Can you work these out from the model? Positions are in its coordinate system, mm. Face numbers are marked on the shaded views. A direction names the side the tool comes from. Give positions to 0.01 mm unless a question says otherwise; leave off trailing zeros. Loops run counter-clockwise (first coordinate to the right, second up) from the corner with the lowest first, then second, coordinate; pieces in that order, holes last. Notation, with made-up numbers: (-12, -20) - (33, -20) arc R19 ccw to (33, -12) - close; hole circle Ø9 at (29, 62). An arc over 180 degrees is marked (long way). Answer in a Markdown table with one row per item.
from build123d import *

# Parameters (mm, degrees)
SKETCH1_W           = 203.2
SKETCH1_H           = 304.8
BOSS_EXTRUDE1_DEPTH = 203.2
SKETCH2_W           = 177.8
SKETCH2_H           = 279.4
CUT_EXTRUDE1_DEPTH  = 190.5
SKETCH3_W           = 7.62
SKETCH3_H           = 101.6
CUT_EXTRUDE2_DEPTH  = 190.5
SKETCH4_R           = 6.35
BOSS_EXTRUDE2_DEPTH = 279.4
BOSS_EXTRUDE3_DEPTH = 25.4
CUT_EXTRUDE3_DEPTH  = 12.7
SKETCH4_2_R         = 6.35
BOSS_EXTRUDE5_DEPTH = 12.7


with BuildPart() as part:
    # Sketch1 → Boss-Extrude1 (new body)
    with BuildSketch(Plane.XY):
        Rectangle(SKETCH1_W, SKETCH1_H)
    extrude(amount=BOSS_EXTRUDE1_DEPTH)

    # Sketch2 → Cut-Extrude1 (cut)
    with BuildSketch(Plane.XY.offset(203.2)):
        Rectangle(SKETCH2_W, SKETCH2_H)
    extrude(amount=-CUT_EXTRUDE1_DEPTH, mode=Mode.SUBTRACT)

    # Sketch3 → Cut-Extrude2 (cut)
    with BuildSketch(Plane(origin=(0, 152.4, 0), x_dir=(1, 0, 0), z_dir=(0, 1, 0))):
        with Locations((0, -101.6)):
            Rectangle(SKETCH3_W, SKETCH3_H)
    extrude(amount=-CUT_EXTRUDE2_DEPTH, mode=Mode.SUBTRACT)

    # Sketch4 → Boss-Extrude2 (add)
    with BuildSketch(Plane(origin=(0, -139.7, 0), x_dir=(1, 0, 0), z_dir=(0, 1, 0))):
        with Locations((-69.85, -63.5)):
            Circle(SKETCH4_R)
        with Locations((69.85, -63.5)):
            Circle(SKETCH4_R)
        with Locations((69.85, -139.7)):
            Circle(SKETCH4_R)
        with Locations((-69.85, -139.7)):
            Circle(SKETCH4_R)
    extrude(amount=BOSS_EXTRUDE2_DEPTH)

    # Sketch7 → Boss-Extrude3 (add)
    with BuildSketch(Plane(origin=(0, -139.7, 0), x_dir=(1, 0, 0), z_dir=(0, 1, 0))):
        with BuildLine():
            Line((-69.85, -53.975), (-60.325, -53.975))
            Line((-60.325, -53.975), (-28.575, -53.975))
            Line((-28.575, -53.975), (-28.575, -149.225))
            Line((-28.575, -149.225), (-60.325, -149.225))
            Line((-60.325, -149.225), (-69.85, -149.225))
            ThreePointArc((-69.85, -149.225), (-79.375, -139.7), (-69.85, -130.175))
            Line((-69.85, -130.175), (-60.325, -130.175))
            Line((-60.325, -130.175), (-60.325, -73.025))
            Line((-60.325, -73.025), (-69.85, -73.025))
            ThreePointArc((-69.85, -73.025), (-79.375, -63.5), (-69.85, -53.975))
        make_face()
        with BuildLine():
            Line((60.325, -53.975), (28.575, -53.975))
            Line((28.575, -53.975), (28.575, -149.225))
            Line((28.575, -149.225), (60.325, -149.225))
            Line((60.325, -149.225), (69.85, -149.225))
            ThreePointArc((69.85, -149.225), (79.375, -139.7), (69.85, -130.175))
            Line((69.85, -130.175), (60.325, -130.175))
            Line((60.325, -130.175), (60.325, -73.025))
            Line((60.325, -73.025), (69.85, -73.025))
            ThreePointArc((69.85, -73.025), (79.375, -63.5), (69.85, -53.975))
            Line((69.85, -53.975), (60.325, -53.975))
        make_face()
    extrude(amount=BOSS_EXTRUDE3_DEPTH)

    # Sketch7_4 → Cut-Extrude3 (cut)
    with BuildSketch(Plane(origin=(0, -139.7, 0), x_dir=(1, 0, 0), z_dir=(0, 1, 0))):
        with BuildLine():
            Line((-69.85, -53.975), (-60.325, -53.975))
            Line((-60.325, -53.975), (-28.575, -53.975))
            Line((-28.575, -53.975), (-28.575, -149.225))
            Line((-28.575, -149.225), (-60.325, -149.225))
            Line((-60.325, -149.225), (-69.85, -149.225))
            ThreePointArc((-69.85, -149.225), (-79.375, -139.7), (-69.85, -130.175))
            Line((-69.85, -130.175), (-60.325, -130.175))
            Line((-60.325, -130.175), (-60.325, -73.025))
            Line((-60.325, -73.025), (-69.85, -73.025))
            ThreePointArc((-69.85, -73.025), (-79.375, -63.5), (-69.85, -53.975))
        make_face()
        with BuildLine():
            Line((60.325, -53.975), (28.575, -53.975))
            Line((28.575, -53.975), (28.575, -149.225))
            Line((28.575, -149.225), (60.325, -149.225))
            Line((60.325, -149.225), (69.85, -149.225))
            ThreePointArc((69.85, -149.225), (79.375, -139.7), (69.85, -130.175))
            Line((69.85, -130.175), (60.325, -130.175))
            Line((60.325, -130.175), (60.325, -73.025))
            Line((60.325, -73.025), (69.85, -73.025))
            ThreePointArc((69.85, -73.025), (79.375, -63.5), (69.85, -53.975))
            Line((69.85, -53.975), (60.325, -53.975))
        make_face()
    extrude(amount=CUT_EXTRUDE3_DEPTH, mode=Mode.SUBTRACT)

    # Sketch4_2 → Boss-Extrude5 (add)
    with BuildSketch(Plane(origin=(0, -139.7, 0), x_dir=(1, 0, 0), z_dir=(0, 1, 0))):
        with Locations((-69.85, -63.5)):
            Circle(SKETCH4_2_R)
        with Locations((69.85, -63.5)):
            Circle(SKETCH4_2_R)
        with Locations((69.85, -139.7)):
            Circle(SKETCH4_2_R)
        with Locations((-69.85, -139.7)):
            Circle(SKETCH4_2_R)
    extrude(amount=BOSS_EXTRUDE5_DEPTH)


solid = part.part
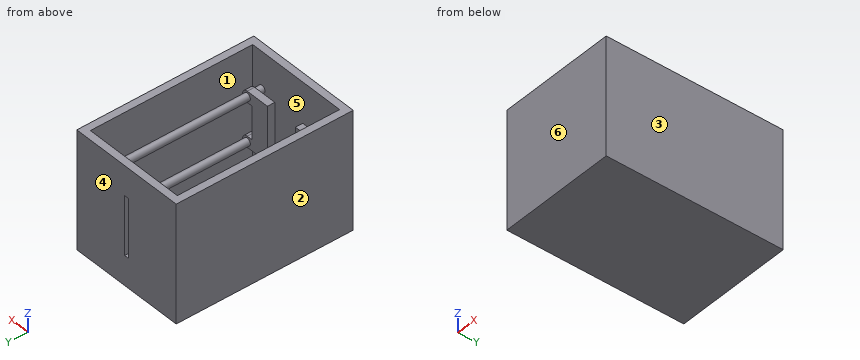
Q1. Imagine slicing it at A-A, the plane x = 43.5. Write out the boundary of the cut face in (y, z) (3 decimals), and give its area (3 significant figures).
Checked values:
| item | result |
|---|---|
| outline | (-152.4, 0) - (152.4, 0) - (152.4, 203.2) - (139.7, 203.2) - (139.7, 12.7) - (-139.7, 12.7) - (-139.7, 203.2) - (-152.4, 203.2) - close; (-127, 53.975) - (-114.3, 53.975) - (-114.3, 149.225) - (-127, 149.225) - close |
| area | 9,920 mm² |
Q2. If we mould it in two halves opening along Y, with no side actions, what happens to the marked faces 3, 4, 5 and 6? For each: released by +Y, released by -Y, zero draft, split by the parting line, or undercut.
Checked values:
| item | result |
|---|---|
| face 3 | zero draft |
| face 4 | released by +Y |
| face 5 | undercut |
| face 6 | released by -Y |
Q3. Imagine slicing it at D-D, the plane x = -14. Write out the boundary of the cut face in (y, z).
Checked values:
| item | result |
|---|---|
| outline | (-152.4, 0) - (152.4, 0) - (152.4, 203.2) - (139.7, 203.2) - (139.7, 12.7) - (-139.7, 12.7) - (-139.7, 203.2) - (-152.4, 203.2) - close |
Q4. On a 3-axis mill with a long thin cutter (end or side, diameter ignored), from which of +Z, -Z, +X, -X, +Y, -Y can I reach the whole of each face in a straight line? I mean the marked faces 1 and 2. Say none if no direction works.
Checked values:
| item | result |
|---|---|
| face 1 | +Z |
| face 2 | +Z, -Z, -X, +Y, -Y |
Q5. If I drill on line 1 (Y direction, x = -71, z = 72.5); line 2 (X direction, y = 104, z = 107.5); line 3 (Y direction, x = -21, z = 117), over which ranges is the centre line in solid material (lowest first)? Write a range as [from, to].
Checked values:
| item | result |
|---|---|
| line 1 | y = [-152.4, -139.7], [-127, -114.3], [139.7, 152.4] |
| line 2 | x = [-101.6, -88.9], [88.9, 101.6] |
| line 3 | y = [-152.4, -139.7], [139.7, 152.4] |
Q6. Imagine slicing it at C-C, the plane y = -30.5. Write out the boundary of the cut face in (x, z), and give its area (3 significant figures).
Checked values:
| item | result |
|---|---|
| outline | (-101.6, 0) - (101.6, 0) - (101.6, 203.2) - (88.9, 203.2) - (88.9, 12.7) - (-88.9, 12.7) - (-88.9, 203.2) - (-101.6, 203.2) - close; circle Ø12.7 at (-69.85, 63.5); circle Ø12.7 at (-69.85, 139.7); circle Ø12.7 at (69.85, 63.5); circle Ø12.7 at (69.85, 139.7) |
| area | 7,930 mm² |
Q7. For pin 1 (6 mm diameter, centred on x = 33, y = 60.5, fed in from +Z); pin 2 (14 mm diameter, centred on x = -59, y = -123.5, fed in from +Z) (3 decimals), each with a flat end and sliding along its axis, tell me the tip position at first contact or that it passes through.
Checked values:
| item | result |
|---|---|
| pin 1 | stops at z = 12.7 |
| pin 2 | stops at z = 149.225 |
Q8. Imagine slicing it at B-B, the plane z = 88.5. Write out the boundary of the cut face in (x, y) (3 decimals).
Checked values:
| item | result |
|---|---|
| outline | (-101.6, -152.4) - (101.6, -152.4) - (101.6, 152.4) - (3.81, 152.4) - (3.81, 139.7) - (88.9, 139.7) - (88.9, -139.7) - (-88.9, -139.7) - (-88.9, 139.7) - (-3.81, 139.7) - (-3.81, 152.4) - (-101.6, 152.4) - close; (-60.325, -127) - (-28.575, -127) - (-28.575, -114.3) - (-60.325, -114.3) - close; (28.575, -127) - (60.325, -127) - (60.325, -114.3) - (28.575, -114.3) - close |
